```python
from build123d import *

# Parameters (mm, degrees)
SKETCH_2_W          = 35
SKETCH_2_H          = 35
EXTRUDE_1_DEPTH     = 5
SKETCH_3_R          = 1.5
SKETCH_3_W          = 11
SKETCH_3_H          = 7.715
CUT_EXTRUDE_1_DEPTH = 26.248762346
SKETCH_4_W          = 5
SKETCH_4_H          = 8
EXTRUDE_2_DEPTH     = 1.5
SKETCH_5_W          = 4
SKETCH_5_H          = 7.5
EXTRUDE_3_DEPTH     = 20
FILLET_1_R          = 3.75
SKETCH_6_R          = 2.15
CUT_EXTRUDE_2_DEPTH = 8
FILLET_2_R          = 2.5
FILLET_3_R          = 2.5
FILLET_4_R          = 1
FILLET_5_R          = 1
FILLET_6_R          = 1


# Some blends are built 0.0001 mm under size
with BuildPart() as part:
    # 草图2 → 凸台-拉伸1 (new body)
    with BuildSketch(Plane(origin=(0, 0, 0), x_dir=(1, 0, 0), z_dir=(0, 1, 0))):
        Rectangle(SKETCH_2_W, SKETCH_2_H)
    extrude(amount=EXTRUDE_1_DEPTH)

    # 草图3 → 切除-拉伸1 (cut, through all)
    with BuildSketch(Plane(origin=(0, 5, 0), x_dir=(1, 0, 0), z_dir=(0, 1, 0))):
        with Locations(Location((-14.285, 14.285, 0), (0, 0, 270))):
            Circle(SKETCH_3_R)
        with Locations(Location((-14.285, -14.285, 0), (0, 0, 90))):
            Circle(SKETCH_3_R)
        with Locations(Location((14.285, -14.285, 0), (0, 0, 270))):
            Circle(SKETCH_3_R)
        with Locations(Location((14.285, 14.285, 0), (0, 0, 90))):
            Circle(SKETCH_3_R)
        with Locations((-6, 13.6425)):
            Rectangle(SKETCH_3_W, SKETCH_3_H)
    extrude(amount=-CUT_EXTRUDE_1_DEPTH, mode=Mode.SUBTRACT)

    # 草图4 → 凸台-拉伸2 (add)
    with BuildSketch(Plane.XZ):
        Rectangle(SKETCH_4_W, SKETCH_4_H)
    extrude(amount=EXTRUDE_2_DEPTH)

    # 草图5 → 凸台-拉伸3 (add)
    with BuildSketch(Plane.XZ.offset(1.5)):
        Rectangle(SKETCH_5_W, SKETCH_5_H)
    extrude(amount=EXTRUDE_3_DEPTH)

    # 圆角1
    fillet_1_edges = [part.edges().sort_by_distance(p)[0] for p in [
        (0, -21.5, -3.75),
        (0, -21.5, 3.75),
    ]]
    fillet(fillet_1_edges, radius=FILLET_1_R - 0.0001)  # a hair under: the kernel refuses the full size

    # 草图6 → 切除-拉伸2 (cut)
    with BuildSketch(Plane.ZY.offset(2)):
        with Locations((0, -17.75)):
            Circle(SKETCH_6_R)
    extrude(amount=-CUT_EXTRUDE_2_DEPTH, mode=Mode.SUBTRACT)

    # 圆角2
    fillet_2_edges = [part.edges().sort_by_distance(p)[0] for p in [
        (17.5, 2.5, 17.5),
        (-17.5, 2.5, 17.5),
        (-17.5, 2.5, -17.5),
        (17.5, 2.5, -17.5),
    ]]
    fillet(fillet_2_edges, radius=FILLET_2_R)

    # 圆角3
    fillet_3_edges = [part.edges().sort_by_distance(p)[0] for p in [
        (-11.5, 2.5, -17.5),
        (-0.5, 2.5, -17.5),
    ]]
    fillet(fillet_3_edges, radius=FILLET_3_R)

    # 圆角4
    fillet_4_edges = [part.edges().sort_by_distance(p)[0] for p in [
        (-14.5, 0, -17.5),
        (-11.5, 0, -12.3925),
        (-12.232233047, 0, -16.767766953),
        (0.232233047, 0, -16.767766953),
        (-0.5, 0, -12.3925),
        (-6, 0, -9.785),
        (8.5, 0, -17.5),
        (17.5, 0, 0),
        (0, 0, 17.5),
        (-17.5, 0, 0),
        (-16.767766953, 0, -16.767766953),
        (-16.767766953, 0, 16.767766953),
        (16.767766953, 0, 16.767766953),
        (16.767766953, 0, -16.767766953),
    ]]
    fillet(fillet_4_edges, radius=FILLET_4_R)

    # 圆角5
    fillet_5_edges = [part.edges().sort_by_distance(p)[0] for p in [
        (2.5, 0, 0),
        (0, 0, 4),
        (-2.5, 0, 0),
        (0, 0, -4),
    ]]
    fillet(fillet_5_edges, radius=FILLET_5_R)

    # 圆角6
    # the kernel refuses this fillet: 1 mm, written as the material it takes off along each edge
    with BuildSketch(Plane(origin=(-3.961914255, -1.5, -4), x_dir=(0, 0.9999810692345785, -0.006153143299889555), z_dir=(1, 0, 0)), Plane(origin=(3.961914255, -1.5, 4), x_dir=(0, 0.9999810692345785, 0.006153143299889555), z_dir=(-1, 0, 0))) as fillet_6_piece_1:
        with BuildLine():
            CenterArc((0.663387726, 0.996904498), FILLET_6_R, 228.323350496, 37.167285461)
            Line((-0.001538286, 0.249995267), (-0.068030887, 0.175304344))
            ThreePointArc((-0.068030887, 0.175304344), (-0.10076725, 0.124382319), (-0.099998107, -0.000615314))
            Line((-0.099998107, -0.000615314), (0.000615314, -0.099998107))
            ThreePointArc((0.000615314, -0.099998107), (0.500605849, -0.096921535), (0.5769035, -0.09969045))
            Line((0.5769035, -0.09969045), (0.584765702, 0))
        make_face()
    extrude(amount=7.923828511, mode=Mode.SUBTRACT)
    with BuildSketch(Plane(origin=(-2.5, -1.5, 5.734079277), x_dir=(-0.027211919166029507, 0.9996296871618517, 0), z_dir=(0, 0, -1)), Plane(origin=(2.5, -1.5, -5.734079277), x_dir=(0.02721191916602949, 0.9996296871618517, 0), z_dir=(0, 0, 1))) as fillet_6_piece_2:
        with BuildLine():
            CenterArc((0.860236658, 0.986023728), FILLET_6_R, 209.091705597, 51.317812547)
            Line((-0.01360596, 0.499814844), (-0.100990221, 0.451193955))
            ThreePointArc((-0.100990221, 0.451193955), (-0.106765949, 0.24718623), (-0.099962969, -0.002721192))
            Line((-0.099962969, -0.002721192), (0.002721192, -0.099962969))
            ThreePointArc((0.002721192, -0.099962969), (0.502536035, -0.086357009), (0.676971216, -0.098602373))
            Line((0.676971216, -0.098602373), (0.693631711, 0))
        make_face()
    extrude(amount=11.468158553, mode=Mode.SUBTRACT)


solid = part.part
```
The model under review builds one solid part; all positions refer to its coordinate system, in mm. A direction names the side the tool comes from. Give positions to 0.01 mm unless a question says otherwise; leave off trailing zeros. Write each loop counter-clockwise with the first axis right and the second up, starting at its lowest first coordinate (ties: lowest second). Pieces come first, ordered by that corner, then holes. Notation, with made-up numbers: M -28,-19 L 5,-19 A15 ccw 5,-2 Z; hole C 84.25,9 d10. An arc over 180 degrees is marked long. Write item = value, one per line. Start each with the question number.
Q1. We need section D-D (x = 5.5). State the section outline as (y, z) points.
Q2. We need section C-C (y = 2). State the section outline as (x, z) points (3 decimals).
Q3. We need section A-A (y = -17.25). State the section outline as (x, z) points, plus the area to 3 significant figures.
Q4. For line 1 (Z direction, x = -14, y = 4); line 2 (X direction, y = 2, z = -12.5); line 3 (Y direction, x = -9.5, z = 10), list the stretches that pass through material, from the lowest coordinate up.
Q5. Mouldability with a two-part tool opening along Z and no side actions: class faces 4 (the face through (-4, 0, 0)), 5 (the face through (13.27, 2.54, -13.18)), 6 (the face through (-14.5, 3, -17.5)) as released by +Z, released by -Z, zero draft, split by the parting line, or undercut.
Q6. Machinability: for faces 1 (the face through (-6, 3, -9.785)), 2 (the face through (-0.199, 0.285, -11.936)), 3 (the face through (-2, -11, 0)), which of the approach directions +Z, -Z, +X, -X, +Y, -Y give a long, thin tool a straight path to every point of the face, cutting with its end or side? Answer none if there is none.
Q7. Clearance check with flat-ended pins moving along their axes: pin 1 (2 mm diameter, centred on y = -6.5, z = -0.5, fed in from -X); pin 2 (3 mm diameter, centred on x = 0, y = -13.5, fed in from -Z); pin 3 (5 mm diameter, centred on x = 14.285, z = 14.285, fed in from -Y); pin 4 (10 mm diameter, centred on x = -8.5, y = -17, fed in from -Z). State where each tip first meets the part, or that it passes through.
Q8. We need section B-B (x = -6.5). State the section outline as (y, z) points (3 decimals).
Result set:
q1.outline = M 0,-16.5 A1 ccw 1,-17.5 L 5,-17.5 L 5,17.5 L 1,17.5 A1 ccw 0,16.5 Z
q2.outline = M -17.5,-15 A2.5 ccw -15,-17.5 L -14,-17.5 A2.5 ccw -11.5,-15 L -11.5,-9.785 L -0.5,-9.785 L -0.5,-15 A2.5 ccw 2,-17.5 L 15,-17.5 A2.5 ccw 17.5,-15 L 17.5,15 A2.5 ccw 15,17.5 L -15,17.5 A2.5 ccw -17.5,15 Z; hole C -14.285,-14.285 d3; hole C -14.285,14.285 d3; hole C 14.285,-14.285 d3; hole C 14.285,14.285 d3
q3.outline = M -2,-3.75 L 2,-3.75 L 2,-2.09 L -2,-2.09 Z; M -2,2.09 L 2,2.09 L 2,3.75 L -2,3.75 Z
q3.area = 13.3 mm2
q4.line_1 = -17.5 to -15.76, -12.81 to 12.81, 15.76 to 17.5
q4.line_2 = -17.5 to -11.5, -0.5 to 17.5
q4.line_3 = 0 to 5
q5.face_4 = zero draft
q5.face_5 = undercut
q5.face_6 = released by -Z
q6.face_1 = -Z, +Y, -Y
q6.face_2 = -Z, -Y
q6.face_3 = +Z, -Z, -X, -Y
q7.pin_1 = -2
q7.pin_2 = -3.75
q7.pin_3 = 0
q7.pin_4 = through
q8.outline = M 0,-8.785 A1 ccw 1,-9.785 L 5,-9.785 L 5,17.5 L 1,17.5 A1 ccw 0,16.5 Z
